```python
from build123d import *

# Parameters (mm, degrees)
BOSS_EXTRUDE1_DEPTH  = 1.5875
M4_CLEARANCE_HOLE1_D = 4.5
SKETCH5_R            = 3.5
CUT_EXTRUDE1_DEPTH   = 4.1750001


with BuildPart() as part:
    # Sketch1 → Boss-Extrude1 (new body, symmetric)
    with BuildSketch(Plane.XY):
        with BuildLine():
            ThreePointArc((-35.147058824, -14.411764706), (-41.911764706, -12.352941176), (-39.852941176, -5.588235294))
            add(Edge.make_bspline(
                [(-39.852941176, -5.588235294), (-25.087835375, 2.313761515), (0, 5.671559621), (25.087835375, 2.313761515), (39.852941176, -5.588235294)],
                knots=[0, 0, 0, 0.375, 0.625, 1, 1, 1], degree=2))
            ThreePointArc((39.852941176, -5.588235294), (41.911764706, -12.352941176), (35.147058824, -14.411764706))
            add(Edge.make_bspline(
                [(-35.147058824, -14.411764706), (-21.787164625, -7.313761515), (0, -4.421559621), (21.787164625, -7.313761515), (35.147058824, -14.411764706)],
                knots=[0, 0, 0, 0.375, 0.625, 1, 1, 1], degree=2))
        make_face()
    extrude(amount=BOSS_EXTRUDE1_DEPTH, both=True)

    # M4 Clearance Hole1 (through all)
    with Locations(Plane.XY.offset(1.5875)):
        with Locations((37.5, -10), (-12.5, -1.111111111), (12.5, -1.111111111)):
            Hole(M4_CLEARANCE_HOLE1_D / 2)

    # Sketch5 → Cut-Extrude1 (cut, through all)
    with BuildSketch(Plane.XY.offset(1.5875)):
        with Locations((-37.5, -10)):
            Circle(SKETCH5_R)
    extrude(amount=-CUT_EXTRUDE1_DEPTH, mode=Mode.SUBTRACT)


solid = part.part
```
Source: CAD feature listing. Evaluate the final solid. Frame: model axes, mm. Give positions to 0.01 mm unless a question says otherwise; leave off trailing zeros. Use a Markdown table: item, result. Add a question column.
(1) Section query A-A (y = 0). Count the separate pieces of the cut face and the enclosed holes in it, then the cut area to 3 significant figures.
(2) Ray query, line 1 (X direction, y = -2.5, z = 0.6); line 2 (X direction, y = -11, z = 0.4); line 3 (Y direction, x = -12.5, z = -0.9). Return the intervals inside material, ascending.
(3) Pull-direction query (X, two-part tool) for faces 1 (the face through (1, -2, -1.588)), 2 (the face through (-10.252, -1.012, -0.022)); classes: +X half, -X half, draft (parallel to the pull), parting line (faces both ways), or undercut.
Checked values:
| question | item | result |
|---|---|---|
| 1 | separate pieces | 3 |
| 1 | enclosed holes | 0 |
| 1 | area | 149 mm^2 |
| 2 | line 1 | -33.57 to -14.27, -10.73 to 10.73, 14.27 to 33.57 |
| 2 | line 2 | -42.4 to -40.85, -34.15 to -28.02, 28.02 to 35.48, 39.52 to 42.4 |
| 2 | line 3 | -6.19 to -3.36, 1.14 to 3.96 |
| 3 | face 1 | draft |
| 3 | face 2 | undercut |
